Verification items for the finished model (mm, model axes). Face numbers are marked on the shaded views. Give positions to 0.01 mm unless a question says otherwise; leave off trailing zeros. Loops run counter-clockwise (first coordinate to the right, second up) from the corner with the lowest first, then second, coordinate; pieces in that order, holes last. Notation, with made-up numbers: M -16.5,73.25 L -4.5,73.25 A10 ccw -4.5,84.25 Z; hole C 52.25,56 d5. An arc over 180 degrees is marked long. Answer in a Markdown table with one row per item.
```python
from build123d import *

# Parameters (mm, degrees)
EXTRUDE083_DEPTH = 9
SKETCH095_R      = 1.85
SKETCH095_W      = 44
SKETCH095_H      = 10
EXTRUDE084_DEPTH = 2
EXTRUDE082_DEPTH = 10


with BuildPart() as extrude083:
    # Sketch094 → Extrude083 (new body)
    with BuildSketch(Plane.XY):
        Polygon((-51, 36), (-47, 40), (42, 40), (46, 36), (46, -17), (42, -21), (-47, -21), (-51, -17), align=None)
        Polygon((-45, 38), (40, 38), (44, 34), (44, -15), (40, -19), (-45, -19), (-49, -15), (-49, 34), align=None, mode=Mode.SUBTRACT)
    extrude(amount=EXTRUDE083_DEPTH)


with BuildPart() as extrude084:
    # Sketch095 → Extrude084 (new body)
    with BuildSketch(Plane.XY):
        with BuildLine():
            Line((57.636039, 57.5), (64, 51.136039))
            Line((64, 51.136039), (64, -51.136039))
            Line((64, -51.136039), (57.636039, -57.5))
            Line((18, -57.5), (57.636039, -57.5))
            Line((18, -62.50002), (18, -57.5))
            ThreePointArc((10, -62.50002), (14, -66.500019), (18, -62.50002))
            Line((10, -62.50002), (10, -57.5))
            Line((-14, -57.5), (10, -57.5))
            Line((-14, -62.50002), (-14, -57.5))
            ThreePointArc((-22, -62.50002), (-18, -66.5), (-14, -62.50002))
            Line((-22, -62.50002), (-22, -57.5))
            Line((-59.661165, -57.5), (-22, -57.5))
            Line((-59.661165, -57.5), (-68.5, -48.661165))
            Line((-68.5, -48.661165), (-68.5, 48.661165))
            Line((-68.5, 48.661165), (-59.661165, 57.5))
            Line((-59.661165, 57.5), (-22, 57.5))
            Line((-22, 62.5), (-22, 57.5))
            ThreePointArc((-14, 62.5), (-18, 66.5), (-22, 62.5))
            Line((-14, 62.5), (-14, 57.5))
            Line((-14, 57.5), (10, 57.5))
            Line((10, 62.5), (10, 57.5))
            ThreePointArc((18, 62.5), (14, 66.5), (10, 62.5))
            Line((18, 62.5), (18, 57.5))
            Line((18, 57.5), (57.636039, 57.5))
        make_face()
        with Locations((-18, 62.5)):
            Circle(SKETCH095_R, mode=Mode.SUBTRACT)
        with Locations((14, 62.5)):
            Circle(SKETCH095_R, mode=Mode.SUBTRACT)
        with Locations((-18, -62.5)):
            Circle(SKETCH095_R, mode=Mode.SUBTRACT)
        with Locations((14, -62.500019)):
            Circle(SKETCH095_R, mode=Mode.SUBTRACT)
        with Locations((-13, -43)):
            Rectangle(SKETCH095_W, SKETCH095_H, mode=Mode.SUBTRACT)
    extrude(amount=EXTRUDE084_DEPTH)


with BuildPart() as fusion033:
    # Sketch093 → Extrude082 (new body)
    with BuildSketch(Plane.XY):
        Polygon((-59.661165, 57.5), (57.636039, 57.5), (64, 51.136039), (64, -51.136039), (57.636039, -57.5), (-59.661165, -57.5), (-68.5, -48.661165), (-68.5, 48.661165), align=None)
        Polygon((-57.161165, 55), (55.136039, 55), (61.5, 48.636039), (61.5, -48.636039), (55.136039, -55), (-57.161165, -55), (-66, -46.161165), (-66, 46.161165), align=None, mode=Mode.SUBTRACT)
    extrude(amount=EXTRUDE082_DEPTH)

    # Fusion033: union Extrude083, Extrude084
    add(extrude083.part)
    add(extrude084.part)


with BuildPart() as fusion033_1:
    # Fusion033 placement: moved
    add(fusion033.part.moved(Location((0, 0, -7))))


solid = fusion033_1.part
```
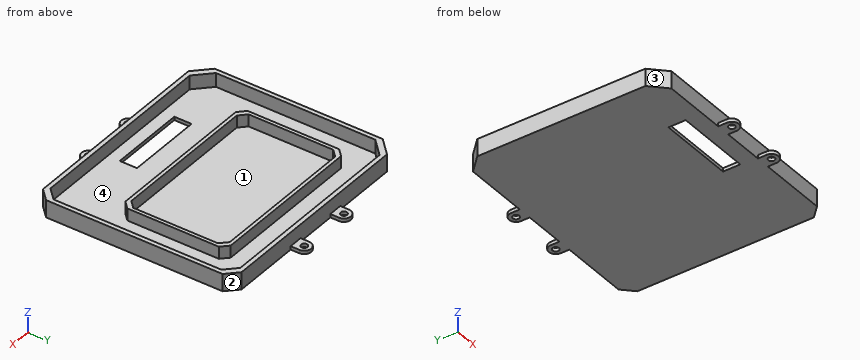
Item 1: Go/stop test with flat-tipped pins: pin 1 (2 mm diameter, centred on x = -12, z = -6.5, fed in from +Y); pin 2 (12 mm diameter, centred on x = -40.5, y = 33, fed in from +Z); pin 3 (2 mm diameter, centred on x = 20, z = 2, fed in from -Y). Record where each tip stops, or that it passes through.
Reported:
| item | result |
|---|---|
| pin 1 | stops at y = 57.5 |
| pin 2 | stops at z = 2 |
| pin 3 | stops at y = -57.5 |
Item 2: Sectioned sample at C-C (y = -41). Record the cut outline in (x, z), and give its area (3 significant figures).
Reported:
| item | result |
|---|---|
| outline | M -68.5,-7 L -35,-7 L -35,-5 L -66,-5 L -66,3 L -68.5,3 Z; M 9,-7 L 64,-7 L 64,3 L 61.5,3 L 61.5,-5 L 9,-5 Z |
| area | 217 mm^2 |
Item 3: Sectioned sample at B-B (x = 14). Record the cut outline in (y, z), and give its area (3 significant figures).
Reported:
| item | result |
|---|---|
| outline | M -66.5,-7 L -64.35,-7 L -64.35,-5 L -66.5,-5 Z; M -60.65,-7 L 60.65,-7 L 60.65,-5 L 57.5,-5 L 57.5,3 L 55,3 L 55,-5 L 40,-5 L 40,2 L 38,2 L 38,-5 L -19,-5 L -19,2 L -21,2 L -21,-5 L -55,-5 L -55,3 L -57.5,3 L -57.5,-5 L -60.65,-5 Z; M 64.35,-7 L 66.5,-7 L 66.5,-5 L 64.35,-5 Z |
| area | 319 mm^2 |
Item 4: Scan lines: L1, parallel to Y at x = -18, z = -5.5; L2, parallel to Y at x = 40, z = -1.5; L3, parallel to Y at x = 14, z = -5.85. Record each from-to range of solid material in increasing order. Write a range as [from, to].
Reported:
| item | result |
|---|---|
| L1 | y = [-66.5, -64.35], [-60.65, -48], [-38, 60.65], [64.35, 66.5] |
| L2 | y = [-57.5, -55], [-21, -19], [38, 40], [55, 57.5] |
| L3 | y = [-66.5, -64.35], [-60.65, 60.65], [64.35, 66.5] |
Item 5: Release check for a two-part mould opening along Y. For the marked faces 1, 2, 3 and 4 record: released by +Y, released by -Y, zero draft, split by the parting line, or undercut.
Reported:
| item | result |
|---|---|
| face 1 | undercut |
| face 2 | released by +Y |
| face 3 | released by -Y |
| face 4 | undercut |
Item 6: Sectioned sample at A-A (z = 0). State how many separate pieces and enclosed holes the cut face has, and give its area (3 significant figures).
Reported:
| item | result |
|---|---|
| separate pieces | 2 |
| enclosed holes | 2 |
| area | 1,830 mm^2 |
